The model under review builds one solid part; all positions refer to its coordinate system, in mm. A direction names the side the tool comes from. Give positions to 0.01 mm unless a question says otherwise; leave off trailing zeros. Loops run counter-clockwise (first coordinate to the right, second up) from the corner with the lowest first, then second, coordinate; pieces in that order, holes last. Notation, with made-up numbers: M 59,80.5 L 74,80.5 A20 ccw 74,100.5 Z; hole C -18.75,70.5 d3. An arc over 180 degrees is marked long. One line per item, written item: value. Start each with the question number.
Q1. We need section A-A on z = 0. Write out the cut boundary in (x, y), plus the area to 3 significant figures.
Q2. We need section B-B on x = 0. Write out the cut boundary in (y, z).
Q3. For pin 1 (1.5 mm diameter, centred on x = -13, y = 11.5, fed in from -Z); pin 2 (3 mm diameter, centred on x = -16.5, y = 18.5, fed in from +Z); pin 3 (8 mm diameter, centred on y = 7.5, z = 1, fed in from +X); pin 4 (1 mm diameter, centred on x = 13, z = 19.5, fed in from -Y), all flat-tipped, find the tip position at first contact; note any pin that passes through.
Q4. We need section C-C on y = 17.25. Write out the cut boundary in (x, z), plus the area to 3 significant figures.
Q5. Mouldability with a two-part tool opening along Z and no side actions: class faces 3 (the face through (-11, 2, -23)), 4 (the face through (25.865, 0.986, -10.724)), 5 (the face through (0, 12, -2)) as released by +Z, released by -Z, zero draft, split by the parting line, or undercut.
Q6. For faces 1 (the face through (23.846, 11.86, 7.509)), 2 (the face through (0, 0, 0)), list the 3-axis set-ups (+Z, -Z, +X, -X, +Y, -Y) from which the entire face can be reached by the end or side of a thin tool; tool diameter is ignored.
Q7. To check wall thickness, follow line 1 along Y through (x, z) = (-9.5, -25); line 2 along Z through (x, y) = (-12.5, 4.5); line 3 along X through (y, z) = (6, 21.5). State the ranges of each line that lie inside material, in increasing order. Write a range as from..to.
Q8. We need section D-D on z = -15. Write out the cut boundary in (x, y), plus the area to 3 significant figures.
Autodesk Fusion 360 part; units mm, degrees
sketch "스케치1" plane through (0, 0, 0) normal (0, 1, 0) x (1, 0, 0)
  circle A0 centre (0, 0) radius 3
  line L0 (-3, 2) -> (3, 2)
  line L1 (3, 2) -> (3, -3)
  line L2 (3, -3) -> (-3, -3)
  line L3 (-3, -3) -> (-3, 2)
  circle A1 centre (0, 0) radius 25
  dimension "d1" = 6
  dimension "d2" = 5
  dimension "d3" = 50
extrude "돌출1" add sketch "스케치1" along normal blind 22 contours A0 L0 | A0 L1 L2 | A0 L0 L1 | A0 L2 L3 | A0 L0 L3 | A1 picked at (2.2415, -0.6297)
sketch "스케치2" plane through (0, 0, 0) normal (0, 1, 0) x (1, 0, 0)
  circle A0 centre (0, 0) radius 28
  dimension "d6" = 56
extrude "돌출2" add sketch "스케치2" along normal blind 2
Solved:
1. outline: M -28,0 L 28,0 L 28,2 L 25,2 L 25,22 L -25,22 L -25,2 L -28,2 Z
1. area: 1,110 mm2
2. outline: M 0,-28 L 2,-28 L 2,-25 L 22,-25 L 22,-3 L 2,-3 L 2,-2 L 22,-2 L 22,25 L 2,25 L 2,28 L 0,28 Z
3. pin 1: z = -21.79
3. pin 2: z = 20
3. pin 3: x = 25
3. pin 4: y = 0
4. outline: C 0,0 d50; hole M -2.24,-2 A3 ccw 2.24,-2 Z
4. area: 1,960 mm2
5. face 3: zero draft
5. face 4: split by the parting line
5. face 5: undercut
6. face 1: +Y
6. face 2: +Z, -Z, +X, -X, -Y
7. line 1: 0..2
7. line 2: -21.65..21.65
7. line 3: -12.76..12.76
8. outline: M -23.64,0 L 23.64,0 L 23.64,2 L 20,2 L 20,22 L -20,22 L -20,2 L -23.64,2 Z
8. area: 895 mm2
